The listing builds one solid part. Answer for the finished solid, in the listing's coordinates (mm). Face numbers are marked on the shaded views. A direction names the side the tool comes from. Give positions to 0.01 mm unless a question says otherwise; leave off trailing zeros. Write each loop counter-clockwise with the first axis right and the second up, starting at its lowest first coordinate (ties: lowest second). Pieces come first, ordered by that corner, then holes. Notation, with made-up numbers: (56, 20.25) -> (84, 20.25) arc R18 cw to (84, 35.25) -> close; hole circle Ø7 at (84.25, -4). An arc over 180 degrees is marked (long way). One line per question, with ' | ' between items.
from build123d import *

# Parameters (mm, degrees)
F1_DEPTH = 25.4


with BuildPart() as f1:
    # F0 (on Front) → F1 (new body)
    with BuildSketch(Plane.XZ):
        Polygon((-5.4805049415, 43.8882187009), (-69.4460719824, 43.8882187009), (-69.4460719824, 17.7506506443), (12.4516431242, 17.7506506443), (12.4516431242, 43.8882187009), align=None)
        with BuildLine():
            ThreePointArc((12.8084794992, 61.8168160262), (-0.1015057146, 56.6937014517), (-5.4805049415, 43.8882187009))
            Line((-5.4805049415, 43.8882187009), (12.4516431242, 43.8882187009))
            Line((12.4516431242, 43.8882187009), (12.4516431242, 58.6995072663))
            ThreePointArc((12.4516431242, 58.6995072663), (12.5411425509, 60.2683401209), (12.8084794992, 61.8168160262))
        make_face()
        with BuildLine():
            ThreePointArc((23.3348449459, 72.183508426), (16.5668649609, 68.5281371373), (12.8084794992, 61.8168160262))
            ThreePointArc((12.8084794992, 61.8168160262), (12.9028776825, 61.8146885604), (12.9972633549, 61.81206407))
            ThreePointArc((12.9972633549, 61.81206407), (16.3462648739, 66.1901444716), (21.6024321989, 67.8502963409))
            Line((21.6024321989, 67.8502963409), (37.4638475478, 67.8502963409))
            Line((37.4638475478, 67.8502963409), (37.4638475478, 73.7137471339))
            ThreePointArc((37.4638475478, 73.7137471339), (30.3592257705, 73.3190682295), (23.3348449459, 72.183508426))
        make_face()
        with BuildLine():
            ThreePointArc((12.9972633549, 61.81206407), (12.9028776825, 61.8146885604), (12.8084794992, 61.8168160262))
            ThreePointArc((12.8084794992, 61.8168160262), (12.5411425509, 60.2683401209), (12.4516431242, 58.6995072663))
            ThreePointArc((12.4516431242, 58.6995072663), (12.5890802771, 60.279516071), (12.9972633549, 61.81206407))
        make_face()
    extrude(amount=F1_DEPTH)


solid = f1.part
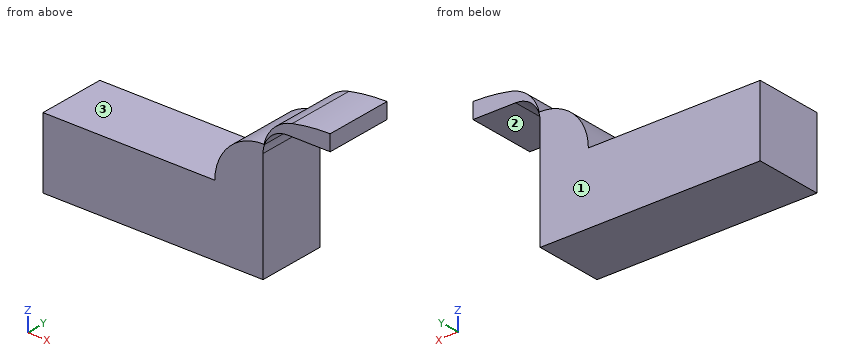
Item 1: Find section A-A (y = -2). Write down the section's boundary in (x, z), then the cut area to 3 significant figures.
Answers below:
outline: (-69.45, 17.75) -> (12.45, 17.75) -> (12.45, 58.7) arc R9.15 cw to (21.6, 67.85) -> (37.46, 67.85) -> (37.46, 73.71) arc R67.94 ccw to (23.33, 72.18) arc R13.79 ccw to (12.81, 61.82) arc R17.93 ccw to (-5.48, 43.89) -> (-69.45, 43.89) -> close | area: 2,500 mm²
Item 2: A tool of negligible diameter and unlimited length cuts with its end or side. For the marked faces 1, 2 and 3, from which of +Z, -Z, +X, -X, +Y, -Y can it reach the whole face along a straight path? Write none if from no direction.
Answers below:
face 1: +Z, -Z, +X, -X, +Y | face 2: -Z, +X, +Y, -Y | face 3: +Z, -X, +Y, -Y
Item 3: Consider line 1 (Z direction, x = -51.5, y = -16); line 2 (X direction, y = -11, z = 25); line 3 (Z direction, x = 6, y = -20). Determine where each line is inside the solid, lowest interval first. Write a range as [from, to].
Answers below:
line 1: [17.75, 43.89] | line 2: [-69.45, 12.45] | line 3: [17.75, 60.62]
Item 4: Find section C-C (z = 28). Write down the section's boundary in (x, y), then the cut area to 3 significant figures.
Answers below:
outline: (-69.45, -25.4) -> (12.45, -25.4) -> (12.45, 0) -> (-69.45, 0) -> close | area: 2,080 mm²
Item 5: Find section B-B (x = -38.5). Write down the section's boundary in (y, z).
Answers below:
outline: (-25.4, 17.75) -> (0, 17.75) -> (0, 43.89) -> (-25.4, 43.89) -> close
Item 6: Flat-ended cylindrical pins translate along their axes: pin 1 (8 mm diameter, centred on x = 23.5, y = -5.5, fed in from -Z); pin 2 (10 mm diameter, centred on y = -6.5, z = 62, fed in from +X); pin 3 (6 mm diameter, centred on x = -46, y = -6.5, fed in from +Z). Find the tip coordinate at first contact, or state that the pin passes through.
Answers below:
pin 1: z = 67.61 | pin 2: x = 17.75 | pin 3: z = 43.89
